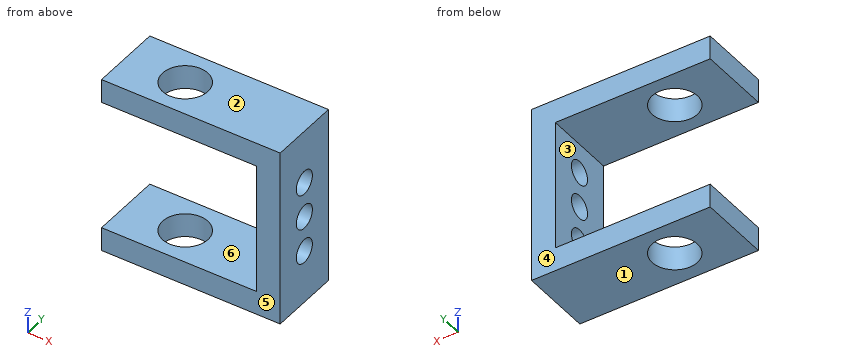
from build123d import *

# Parameters (mm, degrees)
BOSS_EXTRUDE1_DEPTH              = 30
SKETCH3_R                        = 9.5
CUT_EXTRUDE1_DEPTH               = 90
M10X1_0_TAPPED_HOLE1_D           = 9
M10X1_0_TAPPED_HOLE1_DEPTH       = 23
M10X1_0_TAPPED_HOLE1_CBORE_D     = 10
M10X1_0_TAPPED_HOLE1_CBORE_DEPTH = 20
M10X1_0_TAPPED_HOLE1_TIP         = 2.703872786


with BuildPart() as part:
    # Sketch1 → Boss-Extrude1 (new body)
    with BuildSketch(Plane(origin=(0, 0, 0), x_dir=(1, 0, 0), z_dir=(0, 1, 0))):
        Polygon((-55.756575978, -25.748980809), (19.243424022, -25.748980809), (19.243424022, 49.251019191), (-55.756575978, 49.251019191), (-55.756575978, 39.251019191), (9.243424022, 39.251019191), (9.243424022, -15.748980809), (-55.756575978, -15.748980809), align=None)
    extrude(amount=BOSS_EXTRUDE1_DEPTH)

    # Sketch3 → Cut-Extrude1 (cut)
    with BuildSketch(Plane(origin=(0, 0, -49.251019191), x_dir=(-1, 0, 0), z_dir=(0, 0, -1))):
        with Locations((30.756575978, 15)):
            Circle(SKETCH3_R)
    extrude(amount=-CUT_EXTRUDE1_DEPTH, mode=Mode.SUBTRACT)

    # M10x1.0 Tapped Hole1
    with Locations(Plane(origin=(19.243424022, 0, 0), x_dir=(0, 0, -1), z_dir=(1, 0, 0))):
        with Locations((-3.248980809, 15), (11.751019191, 15), (26.751019191, 15)):
            CounterBoreHole(M10X1_0_TAPPED_HOLE1_D / 2, M10X1_0_TAPPED_HOLE1_CBORE_D / 2, M10X1_0_TAPPED_HOLE1_CBORE_DEPTH, depth=M10X1_0_TAPPED_HOLE1_DEPTH)
            with Locations((0, 0, -(M10X1_0_TAPPED_HOLE1_DEPTH + M10X1_0_TAPPED_HOLE1_TIP / 2))):  # 118° drill point
                Cone(0, M10X1_0_TAPPED_HOLE1_D / 2, M10X1_0_TAPPED_HOLE1_TIP, mode=Mode.SUBTRACT)


solid = part.part
Read the model definition and answer for the solid it produces. Units are mm, in the model's axes. Face numbers are marked on the shaded views. A direction names the side the tool comes from. Round coordinates to 2 decimals unless told otherwise and drop trailing zeros. Loops run counter-clockwise (first coordinate to the right, second up) from the corner with the lowest first, then second, coordinate; pieces in that order, holes last. Notation, with made-up numbers: (86.5, 24) - (140.5, 24) arc R25 ccw to (140.5, 63) - close; hole circle Ø10 at (15, 84). An arc over 180 degrees is marked (long way). One line per question, with ' | ' between items. Start each with the question number.
Q1. Flat-ended cylindrical pins translate along their axes: pin 1 (6 mm diameter, centred on y = 15, z = -27.5, fed in from -X); pin 2 (16 mm diameter, centred on y = 15, z = -11.75, fed in from -X). Find the tip coordinate at first contact, or state that the pin passes through.
Q2. Section C-C on x = -28 is taken. Give the vertices of the cut face in (y, z).
Q3. Find the intervals of material crossed by L1, parallel to Z at x = -47, y = 8; L2, parallel to X at y = 25.25, z = -19; L3, parallel to X at y = 21.5, z = 22.5, in increasing order.
Q4. For the marked faces 5 and 6, determine the directions among +Z, -Z, +X, -X, +Y, -Y from which every point of the face is accessible in a straight line to the end or side of a thin tool.
Q5. Section B-B on y = 15 is taken. Give the vertices of the cut face in (x, z).
Q6. For a pull along Z with two mould halves and no side action, classify the marked faces 1, 2, 3 and 4 as +Z half, -Z half, draft (parallel to the pull), parting line (faces both ways), or undercut.
Q7. Section D-D on z = -37.5 is taken. Give the vertices of the cut face in (x, y), plus the area to 3 significant figures.
Q8. Section A-A on x = 3.5 is taken. Give the vertices of the cut face in (y, z), plus the area to 3 significant figures.
Established:
1) pin 1: through | pin 2: x = 9.24
2) outline: (0, -49.25) - (5.91, -49.25) - (5.91, -39.25) - (0, -39.25) - close; (0, 15.75) - (5.91, 15.75) - (5.91, 25.75) - (0, 25.75) - close; (24.09, -49.25) - (30, -49.25) - (30, -39.25) - (24.09, -39.25) - close; (24.09, 15.75) - (30, 15.75) - (30, 25.75) - (24.09, 25.75) - close
3) L1: -49.25 to -39.25, 15.75 to 25.75 | L2: 9.24 to 19.24 | L3: -55.76 to -37.68, -23.83 to 19.24
4) face 5: +Z, -Z, +X, -X, -Y | face 6: -X, +Y, -Y
5) outline: (-55.76, -49.25) - (-40.26, -49.25) - (-40.26, -39.25) - (-55.76, -39.25) - close; (-55.76, 15.75) - (-40.26, 15.75) - (-40.26, 25.75) - (-55.76, 25.75) - close; (-21.26, -49.25) - (19.24, -49.25) - (19.24, -31.75) - (9.24, -31.75) - (9.24, -39.25) - (-21.26, -39.25) - close; (-21.26, 15.75) - (9.24, 15.75) - (9.24, 8.25) - (19.24, 8.25) - (19.24, 25.75) - (-21.26, 25.75) - close; (9.24, -21.75) - (19.24, -21.75) - (19.24, -16.75) - (9.24, -16.75) - close; (9.24, -6.75) - (19.24, -6.75) - (19.24, -1.75) - (9.24, -1.75) - close
6) face 1: -Z half | face 2: +Z half | face 3: undercut | face 4: draft
7) outline: (9.24, 0) - (19.24, 0) - (19.24, 30) - (9.24, 30) - close | area: 300 mm²
8) outline: (0, -49.25) - (30, -49.25) - (30, -39.25) - (0, -39.25) - close; (0, 15.75) - (30, 15.75) - (30, 25.75) - (0, 25.75) - close | area: 600 mm²
